Verification items for the finished model (mm, model axes). A direction names the side the tool comes from. Coordinates: 2 decimals unless noted, no trailing zeros. Order: outer loops, then holes, each group sorted by start corner. A loop starts at its lowest first (then second) coordinate and runs counter-clockwise, first axis right, second up.
Q1. Set-up check for faces 4 (the flat face through (125, 26.547, 6)), 5 (the flat face through (120, -98.453, 7)): record each of +Z, -Z, +X, -X, +Y, -Y from which the full face is reachable in a straight line by a thin tool's end or side.
Q2. Draft check along Y on faces 1 (the flat face through (302.3, -36.2, -0.2)), 2 (the flat face through (120, -99.453, 6)), 3 (the cylindrical face through (233.57, -5.07, -0.51)). Enter one of: pulls with the +Y half, pulls with the -Y half, needs draft (parallel to the pull), parting line crosses it, or undercut.
Q3. Cross-section at A-A, the plane z = 6.75. Record the boundary of the cut face in (x, y), and give its area (3 significant figures).
Q4. Cross-section at C-C, the plane y = -64.5. Record the boundary of the cut face in (x, z).
Q5. Thickness scan on line 1 (Y direction, x = 55.5, z = 1.75); line 2 (Z direction, x = 9.5, y = -57); line 3 (Y direction, x = 162.5, z = -0.25). Record the ranges inside material, lowest first.
Q6. Cross-section at B-B, the plane x = 121. Record the boundary of the cut face in (y, z), and give its area (3 significant figures).
from build123d import *

# Parameters (mm, degrees)
SKETCH_1_W                         = 360
SKETCH_1_H                         = 124
SM_BASE_FLANGE_1_DEPTH             = 1
SM_EDGE_FLANGE_1_STRIP_W           = 6.2
SM_EDGE_FLANGE_1_STRIP_H           = 1
SM_EDGE_FLANGE_1_STRIP_CUT_DEPTH   = 360
SM_EDGE_FLANGE_1_STRIP_2_W         = 6.2
SM_EDGE_FLANGE_1_STRIP_2_H         = 1
SM_EDGE_FLANGE_1_STRIP_CUT_2_DEPTH = 360
SM_EDGE_FLANGE_1_DEPTH             = 360
SM_EDGE_FLANGE_1_BEND_DEPTH        = 360
SKETCH_8_R                         = 11.25
CUT_EXTRUDE_1_DEPTH                = 10


# Sheet-metal steps are written as plain solids
with BuildPart() as part:
    # Sketch 1 → Базовая кромка1 (new body)
    with BuildSketch(Plane.XY):
        with Locations((122.300049421, -36.452668213)):
            Rectangle(SKETCH_1_W, SKETCH_1_H)
    extrude(amount=-SM_BASE_FLANGE_1_DEPTH)

    # Ребро-кромка1 strip (across the edge) → Ребро-кромка1 strip cut (cut)
    with BuildSketch(Plane(origin=(302.300049421, 25.547331787, 0), x_dir=(0, -1, 0), z_dir=(-1, 0, 0))):
        with Locations((-2, -0.5)):
            Rectangle(SM_EDGE_FLANGE_1_STRIP_W, SM_EDGE_FLANGE_1_STRIP_H)
    extrude(amount=SM_EDGE_FLANGE_1_STRIP_CUT_DEPTH, mode=Mode.SUBTRACT)

    # Ребро-кромка1 strip 2 (across the edge) → Ребро-кромка1 strip cut 2 (cut)
    with BuildSketch(Plane(origin=(-57.699950579, -98.452668213, 0), x_dir=(0, 1, 0), z_dir=(1, 0, 0))):
        with Locations((-2, -0.5)):
            Rectangle(SM_EDGE_FLANGE_1_STRIP_2_W, SM_EDGE_FLANGE_1_STRIP_2_H)
    extrude(amount=SM_EDGE_FLANGE_1_STRIP_CUT_2_DEPTH, mode=Mode.SUBTRACT)

    # Ребро-кромка1 section (across the edge) → Ребро-кромка1 (add)
    with BuildSketch(Plane(origin=(302.300049421, 25.547331787, 0), x_dir=(0, -1, 0), z_dir=(-1, 0, 0))):
        with BuildLine():
            Line((-1, 1.1), (-1, 12))
            Line((-1, 12), (0, 12))
            Line((0, 12), (0, 1.1))
            ThreePointArc((0, 1.1), (0.322182541, 0.322182541), (1.1, 0))
            Line((1.1, 0), (1.1, -1))
            ThreePointArc((1.1, -1), (-0.38492424, -0.38492424), (-1, 1.1))
        make_face()
    extrude(amount=SM_EDGE_FLANGE_1_DEPTH)

    # Ребро-кромка1 section 2 (across the edge) → Ребро-кромка1 bend (add)
    with BuildSketch(Plane(origin=(-57.699950579, -98.452668213, 0), x_dir=(0, 1, 0), z_dir=(1, 0, 0))):
        with BuildLine():
            Line((-1, 1.1), (-1, 12))
            Line((-1, 12), (0, 12))
            Line((0, 12), (0, 1.1))
            ThreePointArc((0, 1.1), (0.322182541, 0.322182541), (1.1, 0))
            Line((1.1, 0), (1.1, -1))
            ThreePointArc((1.1, -1), (-0.38492424, -0.38492424), (-1, 1.1))
        make_face()
    extrude(amount=SM_EDGE_FLANGE_1_BEND_DEPTH)

    # Эскиз8 → Вырез-Вытянуть1 (cut)
    with BuildSketch(Plane(origin=(0, 0, -1), x_dir=(-1, 0, 0), z_dir=(0, 0, -1))):
        with Locations((-244.300049421, -8.452668213)):
            Circle(SKETCH_8_R)
        with Locations((-244.300049421, -56.452668213)):
            Circle(SKETCH_8_R)
    extrude(amount=-CUT_EXTRUDE_1_DEPTH, mode=Mode.SUBTRACT)


solid = part.part
Check values:
1. face 4: +Z, -Z, +X, -X, +Y
1. face 5: +Z, +X, -X
2. face 1: needs draft
2. face 2: pulls with the -Y half
2. face 3: undercut
3. outline: (-57.7, -99.45) - (302.3, -99.45) - (302.3, -98.45) - (-57.7, -98.45) - close; (-57.7, 25.55) - (302.3, 25.55) - (302.3, 26.55) - (-57.7, 26.55) - close
3. area: 720 mm2
4. outline: (-57.7, -1) - (236.44, -1) - (236.44, 0) - (-57.7, 0) - close; (252.16, -1) - (302.3, -1) - (302.3, 0) - (252.16, 0) - close
5. line 1: y = -99.45 to -98.45, 25.55 to 26.55
5. line 2: z = -1 to 0
5. line 3: y = -98.96 to 26.06
6. outline: (-99.45, 1.1) arc R2.1 ccw to (-97.35, -1) - (24.45, -1) arc R2.1 ccw to (26.55, 1.1) - (26.55, 12) - (25.55, 12) - (25.55, 1.1) arc R1.1 cw to (24.45, 0) - (-97.35, 0) arc R1.1 cw to (-98.45, 1.1) - (-98.45, 12) - (-99.45, 12) - close
6. area: 149 mm2
